```python
from build123d import *

# Parameters (mm, degrees)
F0_W     = 17
F0_H     = 9
F1_DEPTH = 18
F2_T     = -2
F4_DEPTH = 10


with BuildPart() as f1:
    # F0 (on Top) → F1 (new body)
    with BuildSketch(Plane.XY):
        with Locations((-16.993507, 23.638348)):
            Rectangle(F0_W, F0_H)
    extrude(amount=F1_DEPTH)

    # F2
    f2_openings = [f1.faces().sort_by_distance(p)[0] for p in [
        (-16.993507, 23.638348, 18),
    ]]
    offset(amount=F2_T, openings=f2_openings)

    # F3 (on Top) → F4 (join)
    with BuildSketch(Plane.XY):
        Polygon((-24.837663, 19.885201), (-24.837663, 23.537122), (-29.22078, 23.537122), (-29.22078, 13.90854), (-5.551947, 13.90854), (-5.551947, 23.537122), (-9.35065, 23.537122), (-9.457072, 19.885201), align=None)
        Polygon((-29.22078, 23.537122), (-24.837663, 23.537122), (-24.837663, 28.198052), (-9.35065, 28.198052), (-9.35065, 23.537122), (-5.551947, 23.537122), (-5.551947, 34.918834), (-29.22078, 34.918834), (-29.22078, 28.198052), align=None)
    extrude(amount=F4_DEPTH)


solid = f1.part
```
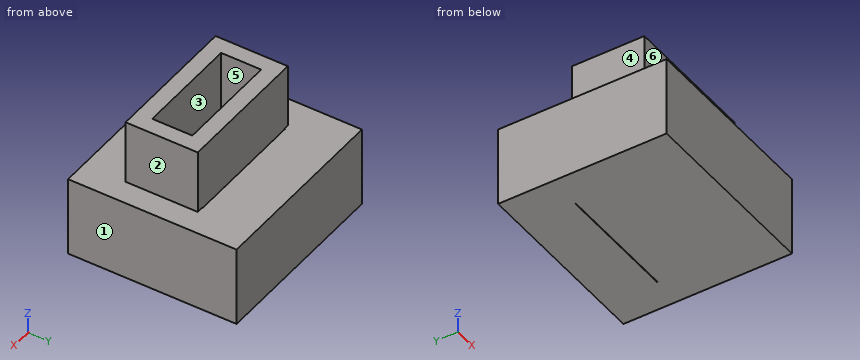
Geometry: final body of the model. Coordinates: model frame, mm. Face numbers are marked on the shaded views. A direction names the side the tool comes from. Round coordinates to 2 decimals unless told otherwise and drop trailing zeros. Loops run counter-clockwise (first coordinate to the right, second up) from the corner with the lowest first, then second, coordinate; pieces in that order, holes last.
Item 1: Section C-C, the plane y = 23.75. Output: boundary loops of the cut face in (x, z), plus the area to 3 significant figures.
Checked values:
outline: (-29.22, 0) - (-5.55, 0) - (-5.55, 10) - (-8.49, 10) - (-8.49, 18) - (-10.49, 18) - (-10.49, 2) - (-23.49, 2) - (-23.49, 18) - (-25.49, 18) - (-25.49, 10) - (-29.22, 10) - close
area: 165 mm2
Item 2: Reachability of the marked faces 1, 2 and 3 from +Z, -Z, +X, -X, +Y, -Y: full face, straight path, thin tool, end or side. Return the list, or none.
Checked values:
face 1: +Z, -Z, +X, +Y, -Y
face 2: +Z, +X, +Y, -Y
face 3: +Z
Item 3: Contact query for flat-ended pins moving along their axis: P1, Ø1.5, axis at x = -18, y = 23.5, coming from the +Z side; P2, Ø2.5, axis at y = 24, z = 14, coming from the +X side; P3, Ø2.5, axis at y = 23, z = 14, coming from the -X side. Output: stop coordinate, or through.
Checked values:
P1: stops at z = 2
P2: stops at x = -8.49
P3: stops at x = -25.49
Item 4: Section B-B, the plane z = 3.5. Output: boundary loops of the cut face in (x, y), plus the area to 3 significant figures.
Checked values:
outline: (-29.22, 13.91) - (-5.55, 13.91) - (-5.55, 34.92) - (-29.22, 34.92) - close; hole (-24.84, 28.14) - (-9.35, 28.14) - (-9.35, 28.2) - (-24.84, 28.2) - close; hole (-23.49, 21.14) - (-10.49, 21.14) - (-10.49, 26.14) - (-23.49, 26.14) - close
area: 431 mm2
Item 5: Line query: L1, parallel to Y at x = -11, z = 16; L2, parallel to Z at x = -8.25, y = 27.5; L3, parallel to X at y = 20.25, z = 13.5. Output: solid intervals per line, ascending.
Checked values:
L1: y = 19.14 to 21.14, 26.14 to 28.14
L2: z = 0 to 10
L3: x = -25.49 to -8.49
Item 6: Section D-D, the plane z = 11.5. Output: boundary loops of the cut face in (x, y).
Checked values:
outline: (-25.49, 19.14) - (-8.49, 19.14) - (-8.49, 28.14) - (-25.49, 28.14) - close; hole (-23.49, 21.14) - (-10.49, 21.14) - (-10.49, 26.14) - (-23.49, 26.14) - close
Item 7: Section A-A, the plane x = -11. Output: boundary loops of the cut face in (y, z).
Checked values:
outline: (13.91, 0) - (28.14, 0) - (28.14, 18) - (26.14, 18) - (26.14, 2) - (21.14, 2) - (21.14, 18) - (19.14, 18) - (19.14, 10) - (13.91, 10) - close; (28.2, 0) - (34.92, 0) - (34.92, 10) - (28.2, 10) - close
Item 8: Mould query, pull axis X, two halves, no side actions, for the marked faces 4, 5 and 6. Classes: released by +X, released by -X, zero draft, split by the parting line, or undercut.
Checked values:
face 4: released by -X
face 5: undercut
face 6: zero draft
